from build123d import *

# Parameters (mm, degrees)
F0_R     = 7.125
F1_DEPTH = 45
F2_R     = 5


with BuildPart() as f1:
    # F0 (on Right) → F1 (new body, symmetric)
    with BuildSketch(Plane.YZ):
        with BuildLine():
            Line((6.666667, 18.856181), (-6.666667, 23.570226))
            ThreePointArc((-6.666667, 23.570226), (-40, 0), (-6.666667, -23.570226))
            Line((-6.666667, -23.570226), (6.666667, -18.856181))
            ThreePointArc((6.666667, -18.856181), (20, 0), (6.666667, 18.856181))
        make_face()
        Circle(F0_R, mode=Mode.SUBTRACT)
    extrude(amount=F1_DEPTH, both=True)

    # F2
    f2_edges = [f1.edges().sort_by_distance(p)[0] for p in [
        (-45, -40, 0),
    ]]
    fillet(f2_edges, radius=F2_R)


solid = f1.part
Could you check a few things on this model? Use its own coordinates, in mm. Give positions to 0.01 mm unless a question says otherwise; leave off trailing zeros. Write each loop counter-clockwise with the first axis right and the second up, starting at its lowest first coordinate (ties: lowest second). Pieces come first, ordered by that corner, then holes. Notation, with made-up numbers: (73.25, 38.5) -> (98.25, 38.5) arc R15 cw to (98.25, 56.5) -> close; hole circle Ø2 at (21.5, 88.25). An arc over 180 degrees is marked (long way). Answer as CSV lines item,"result". Start each with the question number.
(1) I'm going to push flat-ended pins straight in: pin 1 Ø6 at (x, z) = (-26, -11) entering from -Y; pin 2 Ø2 at (x, z) = (22, 5) entering from -Y; pin 3 Ø1 at (x, z) = (3, 4) entering from -Y. Where does each tip first touch, or does it pass through?
(2) Please list where these lines run through material, in increasing order: line 1 (Z direction, x = -9, y = -4); line 2 (Z direction, x = -7, y = 0) (3 decimals); line 3 (Y direction, x = 25, z = 2).
(3) If we section it at A-A, the plane z = 0: Write out the boundary of the cut face in (x, y) (3 decimals), and give its area (3 significant figures).
(4) If we mould it in two halves opening along Y, with no side actions, what happens to faces 1 (the face through (-45, -10, 0)), 2 (the face through (-43.496, -0.382, -19.836)), 3 (the face through (-0.63, 6.58, -2.73))? For each: +Y half, -Y half, draft (parallel to the pull), parting line (faces both ways), or undercut.
(5) If we section it at B-B, the plane x = 27.5: Write out the boundary of the cut face in (y, z) (3 decimals), and give its area (3 significant figures).
Answer list:
1,pin 1,"y = -38.69"
1,pin 2,"y = -39.68"
1,pin 3,"y = -39.75"
2,line 1,"-22.63 to -5.9, 5.9 to 22.63"
2,line 2,"-21.213 to -7.125, 7.125 to 21.213"
2,line 3,"-39.92 to -6.84, 6.84 to 19.9"
3,outline,"(-45, -35) arc R5 ccw to (-40, -40) -> (45, -40) -> (45, -7.125) -> (-45, -7.125) -> close; (-45, 7.125) -> (45, 7.125) -> (45, 20) -> (-40, 20) arc R5 ccw to (-45, 15) -> close"
3,area,"4,110 mm^2"
4,face 1,"draft"
4,face 2,"+Y half"
4,face 3,"undercut"
5,outline,"(-6.667, -23.57) -> (6.667, -18.856) arc R20 ccw to (6.667, 18.856) -> (-6.667, 23.57) arc R25 ccw (long way) to start; hole circle Ø14.25 at (0, 0)"
5,area,"2,160 mm^2"
